Geometry: final body of the model. Coordinates: model frame, mm. Face numbers are marked on the shaded views. Give positions to 0.01 mm unless a question says otherwise; leave off trailing zeros. Order: outer loops, then holes, each group sorted by start corner. A loop starts at its lowest first (then second) coordinate and runs counter-clockwise, first axis right, second up. Notation, with made-up numbers: M -34.5,9.25 L -4.5,9.25 A18 ccw -4.5,41.25 Z; hole C 65,37.25 d2. An arc over 180 degrees is marked long. Use CSV: the item, a comma, the result in double quotes.
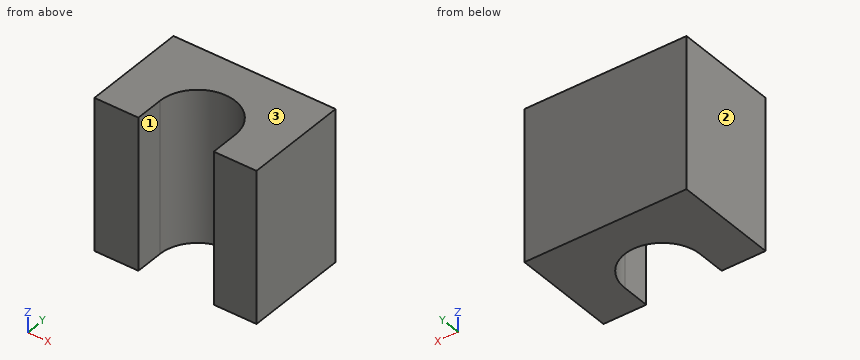
```python
from build123d import *

# Parameters (mm, degrees)
F1_DEPTH = 39


with BuildPart() as f1:
    # F0 (on Top) → F1 (new body)
    with BuildSketch(Plane.XY):
        with BuildLine():
            Line((0, 26.80001), (0, 0))
            Line((0, 0), (11.311256, 0))
            Line((11.311256, 0), (11.311256, 7.377124))
            ThreePointArc((11.311256, 7.377124), (21.105051, 16.979474), (30.690106, 7.168752))
            Line((30.690106, 7.168752), (30.699241, 0))
            Line((30.699241, 0), (41.7, 0))
            Line((41.7, 0), (41.7, 26.80001))
            Line((41.7, 26.80001), (0, 26.80001))
        make_face()
    extrude(amount=F1_DEPTH)


solid = f1.part
```
1. Section A-A, the plane y = 4. Return the cut outline in (x, z).
Answer:
outline,"M 0,0 L 11.31,0 L 11.31,39 L 0,39 Z; M 30.69,0 L 41.7,0 L 41.7,39 L 30.69,39 Z"
2. Section C-C, the plane y = 10. Return the cut outline in (x, z).
Answer:
outline,"M 0,0 L 11.7,0 L 11.7,39 L 0,39 Z; M 30.3,0 L 41.7,0 L 41.7,39 L 30.3,39 Z"
3. Line query: line 1 (X direction, y = 4.5, z = 36.5); line 2 (X direction, y = 15.5, z = 28.5); line 3 (Y direction, x = 25, z = 14). Output: solid intervals per line, ascending.
Answer:
line 1,"0 to 11.31, 30.69 to 41.7"
line 2,"0 to 15.85, 26.15 to 41.7"
line 3,"16.12 to 26.8"
4. Section D-D, the plane x = 24. Return the cut outline in (y, z).
Answer:
outline,"M 16.5,0 L 26.8,0 L 26.8,39 L 16.5,39 Z"
5. Section B-B, the plane z = 6.5. Return the cut outline in (x, y).
Answer:
outline,"M 0,0 L 11.31,0 L 11.31,7.38 A9.69 cw 30.69,7.17 L 30.7,0 L 41.7,0 L 41.7,26.8 L 0,26.8 Z"
6. Pin query (flat end, axial travel): pin 1 Ø12 at (x, y) = (20.5, 16) entering from +Z; pin 2 Ø2 at (x, z) = (19, 13) entering from -Y. Return the tip coordinate at first contact, or that it passes through.
Answer:
pin 1,"z = 39"
pin 2,"y = 16.5"
7. Pull-direction query (X, two-part tool) for the marked faces 1, 2 and 3; classes: +X half, -X half, draft (parallel to the pull), parting line (faces both ways), or undercut.
Answer:
face 1,"undercut"
face 2,"-X half"
face 3,"draft"
